from build123d import *

# Parameters (mm, degrees)
F0_W           = 127.9716864228
F0_H           = 103.479269892
F1_DEPTH       = 25.4
F1_FACE_W      = 127.9716864228
F1_FACE_H      = 103.479269892
F1_FACE1_W     = 127.9716864228
F1_FACE1_H     = 103.479269892
F2_DEPTH       = 76.2
F2_TAPER       = 10
F3_R           = 41.3158420999
F4_DEPTH       = 76.2
F6_D           = 12.7
F6_CBORE_D     = 19.05
F6_CBORE_DEPTH = 12.7
F8_DEPTH       = 101.6
F9_R           = 3.175
F10_R          = 3.175


with BuildPart() as f1:
    # F0 (on Top) → F1 (new body)
    with BuildSketch(Plane.XY):
        with Locations((-2.9518865049, -0.0131409615)):
            Rectangle(F0_W, F0_H)
    extrude(amount=F1_DEPTH)

    # F1_face (on face) + F1_face1 (on face) → F2 (join)
    with BuildSketch(Plane(origin=(-2.9518865049, -0.0131409615, 25.4), x_dir=(1, 0, 0), z_dir=(0, 0, 1))):
        Rectangle(F1_FACE_W, F1_FACE_H)
    with BuildSketch(Plane(origin=(-2.9518865049, -0.0131409615, 0), x_dir=(1, 0, 0), z_dir=(0, 0, -1))):
        Rectangle(F1_FACE1_W, F1_FACE1_H)
    extrude(amount=F2_DEPTH, taper=F2_TAPER, dir=(0, 0, 1))

    # F3 (on Right) → F4 (cut, symmetric)
    with BuildSketch(Plane.YZ):
        with Locations((-1.9303264562, 0)):
            Circle(F3_R)
    extrude(amount=F4_DEPTH, both=True, mode=Mode.SUBTRACT)

    # F6 (through all)
    with Locations(Plane.XY.offset(101.6)):
        with Locations((0, 0)):
            CounterBoreHole(F6_D / 2, F6_CBORE_D / 2, F6_CBORE_DEPTH)

    # F7 (on face) → F8 (join)
    with BuildSketch(Plane.XY.offset(101.6)):
        with BuildLine():
            Line((47.5978407765, -38.3166599775), (-53.5016137863, -38.3166599775))
            Line((-53.5016137863, -38.3166599775), (-30.4048839763, -69.3022799435))
            ThreePointArc((-30.4048839763, -69.3022799435), (-27.0403296326, -72.122907664), (-22.7680607757, -73.1347799301))
            Line((-22.7680607757, -73.1347799301), (22.4154582076, -73.1347799301))
            ThreePointArc((22.4154582076, -73.1347799301), (27.2213525546, -71.8334655106), (30.7140753293, -68.2850958411))
            Line((30.7140753293, -68.2850958411), (47.5978407765, -38.3166599775))
        make_face()
    extrude(amount=-F8_DEPTH)

    # F9
    f9_edges = [f1.edges().sort_by_distance(p)[0] for p in [
        (43.812988, -45.034718, 63.5),
        (40.028135, -51.752776, 12.7),
    ]]
    fillet(f9_edges, radius=F9_R)

    # F10
    f10_edges = [f1.edges().sort_by_distance(p)[0] for p in [
        (-48.493963, -45.034718, 63.5),
        (-43.486312, -51.752776, 12.7),
    ]]
    fillet(f10_edges, radius=F10_R)


solid = f1.part
Geometry check sheet. Reference: the model listing, model coordinates, mm. A direction names the side the tool comes from. Give positions to 0.01 mm unless a question says otherwise; leave off trailing zeros. Write each loop counter-clockwise with the first axis right and the second up, starting at its lowest first coordinate (ties: lowest second). Pieces come first, ordered by that corner, then holes. Notation, with made-up numbers: M 65.5,28 L 80.5,28 A5 cw 80.5,32 Z; hole C 76.5,34 d8. An arc over 180 degrees is marked long. One line per question, with ' | ' between items.
1. Cross-section at D-D (y = 29). Enter the section's corners in (x, z), plus the area to 3 significant figures.
Ans:
outline: M -66.59,27.39 L 60.68,27.39 L 47.6,101.6 L -53.5,101.6 Z | area: 8,470 mm2
2. Mould release check, pull along X, two halves, no side actions. Record for faces 5 (the face through (-48.71, -45.306, 64.003)), 6 (the face through (1.38, -6.2, 64.35)), 7 (the face through (-55.874, -48.367, 44.6)), 8 (the face through (-7.559, -5.796, 95.339)): released by +X, released by -X, zero draft, split by the parting line, or undercut.
Ans:
face 5: released by -X | face 6: undercut | face 7: zero draft | face 8: undercut
3. Gauge pin test, flat ends, axial feed: pin 1 (9.5 mm diameter, centred on x = 4.5, y = 1.5, fed in from +Z); pin 2 (12 mm diameter, centred on x = 37, y = -15.5, fed in from -Z); pin 3 (5 mm diameter, centred on y = -50, z = 68.5, fed in from +X); pin 4 (5 mm diameter, centred on y = -34.5, z = 17.5, fed in from -X). Record the tip position at first contact, or that the pin passes through.
Ans:
pin 1: z = 88.9 | pin 2: z = 36.39 | pin 3: x = 42.42 | pin 4: through
4. Scan lines: line 1 along Y through (x, z) = (0, 97) (3 decimals); line 2 along Y through (x, z) = (0, 97.5) (3 decimals); line 3 along X through (y, z) = (-4, 48). Record each from-to range of solid material in increasing order. Write a range as from..to.
Ans:
line 1: -73.135..-9.525, 9.525..39.101 | line 2: -73.135..-9.525, 9.525..39.013 | line 3: -62.95..-4.93, 4.93..57.05
5. Cross-section at B-B (x = -15). Enter the section's corners in (y, z), plus the area to 3 significant figures.
Ans:
outline: M -73.13,0 L -38.32,0 L -38.32,19.57 A41.32 cw 39.39,0 L 51.73,0 L 51.73,25.4 L 38.29,101.6 L -73.13,101.6 Z | area: 9,560 mm2
6. Cross-section at A-A (y = 0). Enter the section's corners in (x, z) (3 decimals), plus the area to 3 significant figures.
Ans:
outline: M -64.139,41.271 L -6.35,41.271 L -6.35,88.9 L -9.525,88.9 L -9.525,101.6 L -53.502,101.6 Z; M 6.35,41.271 L 58.236,41.271 L 47.598,101.6 L 9.525,101.6 L 9.525,88.9 L 6.35,88.9 Z | area: 5,890 mm2
7. Set-up check for faces 1 (the face through (51, -51.753, 13)), 2 (the face through (-3.85, 45.1, 62.97)), 3 (the face through (51.61, -48.44, 44.18)), 4 (the face through (-56, -51.753, 13)): record each of +Z, -Z, +X, -X, +Y, -Y from which the full face is reachable in a straight line by a thin tool's end or side.
Ans:
face 1: +Z, -Z, +X, -Y | face 2: +Z, +X, -X, +Y | face 3: +Z, +X, -Y | face 4: +Z, -Z, -X, -Y
